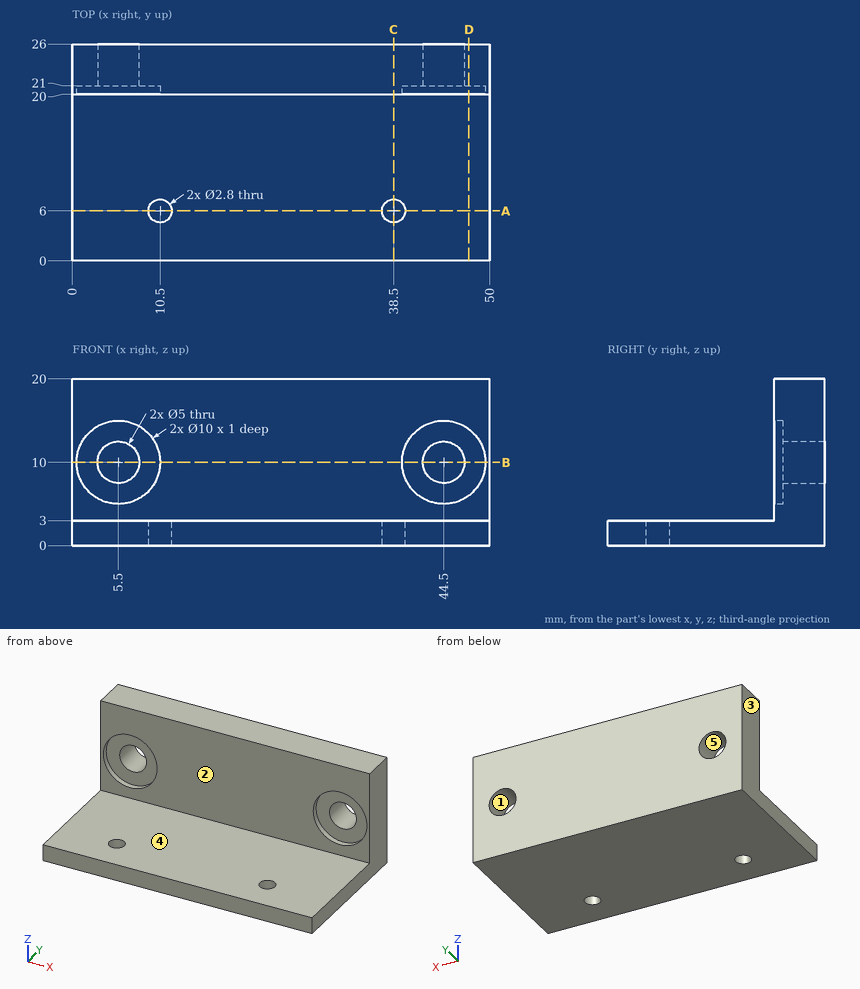
Job drawing, mm, ordinate dimensions from the low corner. One solid piece. A direction names the side the tool comes from. Coordinates: 2 decimals unless noted, no trailing zeros. Order: outer loops, then holes, each group sorted by start corner. A loop starts at its lowest first (then second) coordinate and runs counter-clockwise, first axis right, second up. Notation, with made-up numbers: M 53.5,-15 L 79.5,-15 A10 cw 79.5,0 Z; hole C 21.25,4 d2. An arc over 180 degrees is marked long. Answer as CSV lines item,"result".
(1) Band-saw the part on D-D, the plane x = 47.5. List the corners of the cut face in (y, z).
Geometry says:
outline,"M 0,0 L 26,0 L 26,20 L 20,20 L 20,14 L 21,14 L 21,6 L 20,6 L 20,3 L 0,3 Z"
(2) Wall check: line 1 along X through (y, z) = (6, 2.2); line 2 along Y through (x, z) = (38.5, 1.45); line 3 along Z through (x, y) = (44.5, 20.4). Give the ranges that are in metal, low to high.
Geometry says:
line 1,"x = 0 to 9.1, 11.9 to 37.1, 39.9 to 50"
line 2,"y = 0 to 4.6, 7.4 to 26"
line 3,"z = 0 to 5, 15 to 20"
(3) 3-axis set-ups, long thin cutter, end or side, ignore diameter. For the marked faces 1 and 2: which of +Z, -Z, +X, -X, +Y, -Y reach the whole face in a straight line?
Geometry says:
face 1,"+Y, -Y"
face 2,"+Z, +X, -X, -Y"
(4) Flat gauge pins, fed straight in: pin 1 (2.5 mm diameter, centred on x = 38.5, y = 6, fed in from -Z); pin 2 (10 mm diameter, centred on x = 31, z = 15.5, fed in from -Y); pin 3 (1.5 mm diameter, centred on x = 19, y = 9.5, fed in from +Z). Where does each tip first touch, or does it go through?
Geometry says:
pin 1,"passes through"
pin 2,"stops at y = 20"
pin 3,"stops at z = 3"
(5) Band-saw the part on B-B, the plane z = 10. List the corners of the cut face in (x, y).
Geometry says:
outline,"M 0,20 L 0.5,20 L 0.5,21 L 3,21 L 3,26 L 0,26 Z; M 8,21 L 10.5,21 L 10.5,20 L 39.5,20 L 39.5,21 L 42,21 L 42,26 L 8,26 Z; M 47,21 L 49.5,21 L 49.5,20 L 50,20 L 50,26 L 47,26 Z"
(6) Pull direction X, two halves, no side cores. Call the marked faces 3, 4 and 5: +X half, -X half, draft (parallel to the pull), parting line (faces both ways), or undercut.
Geometry says:
face 3,"-X half"
face 4,"draft"
face 5,"undercut"
(7) Band-saw the part on A-A, the plane y = 6. List the corners of the cut face in (x, z), then the cut area to 3 significant figures.
Geometry says:
outline,"M 0,0 L 9.1,0 L 9.1,3 L 0,3 Z; M 11.9,0 L 37.1,0 L 37.1,3 L 11.9,3 Z; M 39.9,0 L 50,0 L 50,3 L 39.9,3 Z"
area,"133 mm2"
(8) Band-saw the part on C-C, the plane x = 38.5. List the corners of the cut face in (y, z).
Geometry says:
outline,"M 0,0 L 4.6,0 L 4.6,3 L 0,3 Z; M 7.4,0 L 26,0 L 26,20 L 20,20 L 20,3 L 7.4,3 Z"
